Read the model definition and answer for the solid it produces. Units are mm, in the model's axes. Coordinates: 2 decimals unless noted, no trailing zeros. Loops run counter-clockwise (first coordinate to the right, second up) from the corner with the lowest first, then second, coordinate; pieces in that order, holes last. Notation, with made-up numbers: (84, 20) - (137, 20) arc R28 cw to (137, 42) - close; hole circle Ø1 at (72.5, 58.5). An arc over 180 degrees is marked (long way). One line per question, with ' | ' between items. Start each with the question number.
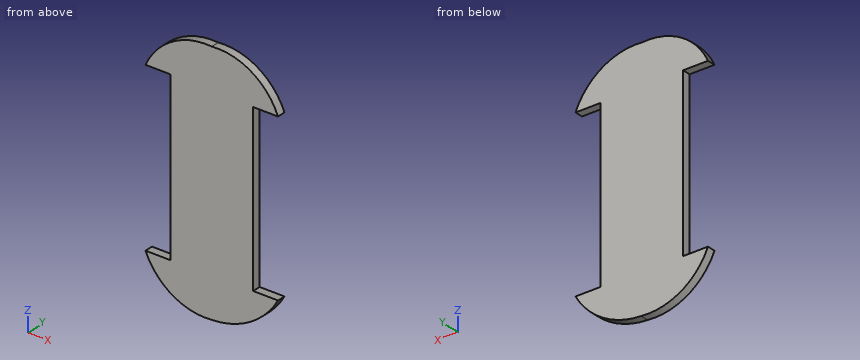
```python
from build123d import *

# Parameters (mm, degrees)
BOSS_EXTRUDE2_DEPTH = 10


with BuildPart() as part:
    # Sketch1 → Boss-Extrude2 (new body)
    with BuildSketch(Plane(origin=(0, 0, 0), x_dir=(1, 0, 0), z_dir=(0, 1, 0))):
        with BuildLine():
            Line((50, 100), (50, -100))
            Line((50, -100), (80, -100))
            ThreePointArc((80, -100), (48.035495612, -137.511232206), (0, -148.53))
            ThreePointArc((0, -148.53), (-47.534227524, -137.586137939), (-80, -101.182229899))
            Line((-80, -101.182229899), (-50, -101.182229899))
            Line((-50, -101.182229899), (-50, 100.833366542))
            Line((-50, 100.833366542), (-80, 100.833366542))
            ThreePointArc((-80, 100.833366542), (-47.524044038, 138.098471025), (0.795654444, 148.518762113))
            ThreePointArc((0.795654444, 148.518762113), (46.745634315, 134.621844661), (80, 100))
            Line((80, 100), (50, 100))
        make_face()
    extrude(amount=BOSS_EXTRUDE2_DEPTH)


solid = part.part
```
1) The part is cut by section D-D on z = 121. Write down the section's boundary in (x, y).
2) Given pin 1 Ø1.5 at (x, y) = (-10.5, 3.5) entering from +Z; pin 2 Ø1.5 at (y, z) = (9, 46.5) entering from +X; pin 3 Ø6 at (x, y) = (-1.5, 2.5) entering from +Z; pin 4 Ø1.5 at (x, z) = (-52, 76.5) entering from +Y, each flat-ended and moving along its own axis, determine where each tip first touches the part or whether it passes through.
3) Find the intervals of material crossed by line 1 along X through (y, z) = (1.5, -65.5); line 2 along Z through (x, y) = (-51.5, 5.75); line 3 along Z through (x, y) = (55, 0.75), in increasing order. Write a range as from..to.
4) The part is cut by section A-A on x = -69. Write down the section's boundary in (y, z), and give its area (3 significant figures).
5) The part is cut by section C-C on z = -73.5. Write down the section's boundary in (x, y).
6) The part is cut by section B-B on y = 8.5. Write down the section's boundary in (x, z).
Answer below:
1) outline: (-67.39, 0) - (67.32, 0) - (67.32, 10) - (-67.39, 10) - close
2) pin 1: z = 148.74 | pin 2: x = 50 | pin 3: z = 148.77 | pin 4: through
3) line 1: -50..50 | line 2: -135.59..-100.83, 101.18..135.08 | line 3: -128.94..-100, 100..132.76
4) outline: (0, -119.42) - (10, -119.42) - (10, -100.83) - (0, -100.83) - close; (0, 101.18) - (10, 101.18) - (10, 119.08) - (0, 119.08) - close | area: 365 mm2
5) outline: (-50, 0) - (50, 0) - (50, 10) - (-50, 10) - close
6) outline: (-80, -100.83) arc R78.38 ccw to (0.8, -148.52) arc R94.82 ccw to (80, -100) - (50, -100) - (50, 100) - (80, 100) arc R78.38 ccw to (0, 148.53) arc R80.42 ccw to (-80, 101.18) - (-50, 101.18) - (-50, -100.83) - close
